Geometry: final body of the model. Coordinates: model frame, mm. A direction names the side the tool comes from. Coordinates: 2 decimals unless noted, no trailing zeros. Order: outer loops, then holes, each group sorted by start corner. A loop starts at its lowest first (then second) coordinate and runs counter-clockwise, first axis right, second up. Notation, with made-up numbers: M 6.25,-32 L 22.25,-32 A15 ccw 22.25,-23 Z; hole C 51,-29.5 d11. An arc over 180 degrees is marked long. Write item = value, one per line.
from build123d import *

# Parameters (mm, degrees)
BASE_FLANGE1_DEPTH    = 6.35
M6X1_0_TAPPED_HOLE1_D = 5
CHAMFER1_SIZE         = 31.75
CHAMFER1_SIZE2        = 18.330871047
EXTRUDE1_REACH        = 170.395
SKETCH5_W             = 4.7752
SKETCH5_H             = 19.05
FILLET1_R             = 6.35
FILLET2_R             = 50.8
FILLET3_R             = 9.525


# Sheet-metal steps are written as plain solids
with BuildPart() as part:
    # Sketch1 → Base-Flange1 (new body)
    with BuildSketch(Plane.XY):
        Polygon((-88.9, 9.525), (69.85, 9.525), (69.85, 142.875), (88.9, 142.875), (88.9, 9.525), (88.9, -9.525), (-88.9, -9.525), align=None)
    extrude(amount=BASE_FLANGE1_DEPTH)

    # M6x1.0 Tapped Hole1 (through all)
    with Locations(Plane.XY.offset(6.35)):
        with Locations((-76.2, 0), (44.45, 0)):
            Hole(M6X1_0_TAPPED_HOLE1_D / 2)

    # Chamfer1
    chamfer1_edges = [part.edges().sort_by_distance(p)[0] for p in [
        (88.9, -9.525, 3.175),
    ]]
    chamfer1_side = [part.faces().sort_by_distance(p)[0] for p in [
        (0, -9.525, 3.175),
    ]]
    chamfer(chamfer1_edges, length=CHAMFER1_SIZE, length2=CHAMFER1_SIZE2, reference=chamfer1_side[0])

    # Sketch5 → Extrude1 (cut, up to next)
    with BuildSketch(Plane.XY.offset(6.35), mode=Mode.PRIVATE) as extrude1_sk1:
        with Locations((-86.5124, 0)):
            Rectangle(SKETCH5_W, SKETCH5_H)
    extrude1_tool1 = extrude(extrude1_sk1.sketch, amount=-EXTRUDE1_REACH, mode=Mode.PRIVATE) & part.part
    add(extrude1_tool1.solids().sort_by_distance((-86.5124, 0, 6.35))[0], mode=Mode.SUBTRACT)

    # Fillet1
    fillet1_edges = [part.edges().sort_by_distance(p)[0] for p in [
        (69.85, 142.875, 3.175),
        (88.9, 142.875, 3.175),
        (-84.1248, 9.525, 3.175),
        (-84.1248, -9.525, 3.175),
    ]]
    fillet(fillet1_edges, radius=FILLET1_R)

    # Fillet2
    fillet2_edges = [part.edges().sort_by_distance(p)[0] for p in [
        (69.85, 9.525, 3.175),
    ]]
    fillet(fillet2_edges, radius=FILLET2_R)

    # Fillet3
    fillet3_edges = [part.edges().sort_by_distance(p)[0] for p in [
        (88.9, 8.805871047, 3.175),
        (57.15, -9.525, 3.175),
    ]]
    fillet(fillet3_edges, radius=FILLET3_R)


solid = part.part
1) Mould query, pull axis Y, two halves, no side actions, for faces 1 (the face through (79, 142.875, 3)), 2 (the face through (69.85, 98, 3)), 3 (the face through (46.948, 0.11, 3.131)), 4 (the face through (-74.2, -1.5, 3.1)). Classes: pulls with the +Y half, pulls with the -Y half, needs draft (parallel to the pull), parting line crosses it, or undercut.
Numbers:
face_1 = pulls with the +Y half
face_2 = needs draft
face_3 = undercut
face_4 = undercut
2) Section B-B, the plane x = 44.45. Return loops of the section in (y, z) (3 decimals).
Numbers:
outline = M -9.525,0 L -2.5,0 L -2.5,6.35 L -9.525,6.35 Z; M 2.5,0 L 16.331,0 L 16.331,6.35 L 2.5,6.35 Z
3) Pin query (flat end, axial travel): pin 1 (3 mm diameter, centred on x = 27, z = 1, fed in from +Y); pin 2 (1.9 mm diameter, centred on x = -21.5, z = 1.5, fed in from +Y) (3 decimals). Return the tip coordinate at first contact, or that it passes through.
Numbers:
pin_1 = 10.41
pin_2 = 9.525
4) Section C-C, the plane y = 0. Return loops of the section in (x, z), and give its area (3 significant figures).
Numbers:
outline = M -84.12,0 L -78.7,0 L -78.7,6.35 L -84.12,6.35 Z; M -73.7,0 L 41.95,0 L 41.95,6.35 L -73.7,6.35 Z; M 46.95,0 L 73.65,0 L 73.65,6.35 L 46.95,6.35 Z
area = 938 mm²
5) Section D-D, the plane y = 67. Return loops of the section in (x, z).
Numbers:
outline = M 69.85,0 L 88.9,0 L 88.9,6.35 L 69.85,6.35 Z
6) Section A-A, the plane z = 2.75. Give the number of separate pieces and of enclosed holes in the cut face, and give its area (3 significant figures).
Numbers:
separate_pieces = 1
enclosed_holes = 2
area = 6,020 mm²
7) Set-up query: faces 5 (the face through (-11, -9.525, 3)), 6 (the face through (-30, 9.525, 3)). Return all of +Z, -Z, +X, -X, +Y, -Y with unobstructed straight access to the full face (end or side cutting, diameter ignored); none if empty.
Numbers:
face_5 = +Z, -Z, +X, -X, -Y
face_6 = +Z, -Z, -X, +Y
8) Line query: L1, parallel to Y at x = -76.2, z = 2.5 (3 decimals); L2, parallel to Y at x = -69, z = 0.5 (3 decimals); L3, parallel to Y at x = 44.45, z = 5.25 (3 decimals). Output: solid intervals per line, ascending.
Numbers:
L1 = -9.525 to -2.5, 2.5 to 9.525
L2 = -9.525 to 9.525
L3 = -9.525 to -2.5, 2.5 to 16.331
